Work out the finished part from the listing and answer in its coordinate system (mm). Face numbers are marked on the shaded views. A direction names the side the tool comes from. Round coordinates to 2 decimals unless told otherwise and drop trailing zeros. Loops run counter-clockwise (first coordinate to the right, second up) from the corner with the lowest first, then second, coordinate; pieces in that order, holes last. Notation, with made-up numbers: (13, 4.25) - (59, 4.25) arc R23 cw to (59, 31.25) - close; hole circle Ø11 at (-38.5, 6). An arc over 180 degrees is marked (long way). Answer as CSV lines item,"result". Start each with the question number.
Q1. Straight lines are drawn through the part: L1, parallel to Z at x = 0, y = 2.5; L2, parallel to Y at x = 5, z = -12.5; L3, parallel to Z at x = -20.5, y = 3. For each, find the intervals that lie inside material, in ascending order. Write a range as [from, to].
Q2. Section C-C on y = 12.75 is taken. Write down the section's boundary in (x, z).
Q3. For the marked faces 1 and 2, determine the directions among +Z, -Z, +X, -X, +Y, -Y from which every point of the face is accessible in a straight line to the end or side of a thin tool.
Q4. Section A-A on z = 0 is taken. Write down the section's boundary in (x, y), then the cut area to 3 significant figures.
Q5. The mould has two halves that part along Z. Classify the marked faces 3, 4 and 5: +Z half, -Z half, draft (parallel to the pull), parting line (faces both ways), or undercut.
Q6. Each of these flat-tipped pins is pushed along its axis until it touches: pin 1 Ø6 at (x, y) = (-10, 9) entering from -Z; pin 2 Ø5 at (x, y) = (-9.5, 3.5) entering from +Z; pin 3 Ø2.5 at (x, z) = (-16.5, 0) entering from -Y; pin 4 Ø3 at (x, y) = (-11, 6) entering from +Z. Where does it stop, or does it pass through?
Q7. Section B-B on x = 0 is taken. Write down the section's boundary in (y, z), then the cut area to 3 significant figures.
Q8. Section D-D on z = -16.5 is taken. Write down the section's boundary in (x, y).
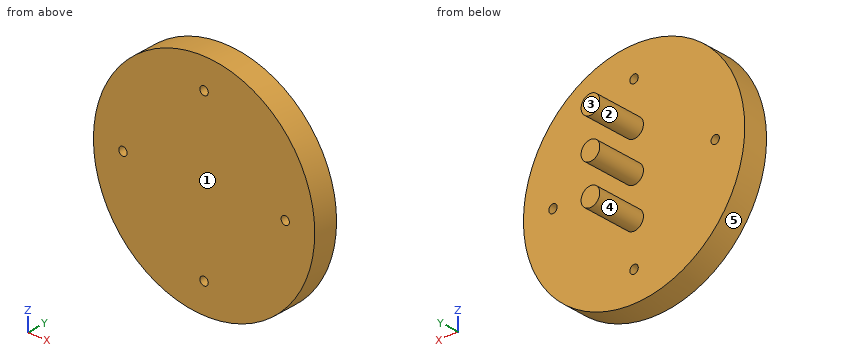
Autodesk Inventor part; units mm, degrees
ref_plane "YZ Plane" through (0, 0, 0) normal (1, 0, 0) x (0, 1, 0)
ref_plane "XZ Plane" through (0, 0, 0) normal (0, 1, 0) x (-1, 0, 0)
ref_plane "XY Plane" through (0, 0, 0) normal (0, 0, 1) x (1, 0, 0)
sketch "Sketch1" plane through (0, 0, 0) normal (0, 1, 0) x (-1, 0, 0)
  circle A0 centre (0, 0) radius 22.5
  dimension "d0" = 45
extrude "Extrusion1" add sketch "Sketch1" along normal blind 5
sketch "Sketch2" plane through (0, 5, 0) normal (0, 1, 0) x (1, 0, 0)
  line L0 (0, 0) -> (0, 8) construction
  line L1 (0, 0) -> (0, -8) construction
  circle A0 centre (0, 8) radius 1.9
  circle A1 centre (0, 0) radius 1.9
  circle A2 centre (0, -8) radius 1.9
  dimension "d3" = 8
  dimension "d4" = 8
  dimension "d5" = 3.8
  dimension "d6" = 3.8
  dimension "d7" = 3.8
extrude "Extrusion2" add sketch "Sketch2" along normal blind 10
sketch "Sketch7" plane through (0, 0, 0) normal (0, -1, 0) x (1, 0, 0)
  circle A0 centre (0, 0) radius 16.5 construction
  circle A1 centre (0, 16.5) radius 0.85
  circle A2 centre (16.5, 0) radius 0.85
  circle A3 centre (-16.5, 0) radius 0.85
  circle A4 centre (0, -16.5) radius 0.85
  dimension "d42" = 33
  dimension "d43" = 1.7
  dimension "d44" = 1.7
  dimension "d45" = 1.7
  dimension "d46" = 1.7
extrude "Extrusion6" cut sketch "Sketch7" against normal blind 5
properties part number "Motor Mount Barebones"
Findings:
1,L1,"z = [-22.5, -17.35], [-15.65, 15.65], [17.35, 22.5]"
1,L2,"y = [0, 5]"
1,L3,"z = [-9.27, 9.27]"
2,outline,"circle Ø3.8 at (0, -8); circle Ø3.8 at (0, 0); circle Ø3.8 at (0, 8)"
3,face 1,"+Z, -Z, +X, -X, -Y"
3,face 2,"+Y"
4,outline,"(-22.5, 0) - (-17.35, 0) - (-17.35, 5) - (-22.5, 5) - close; (-15.65, 0) - (15.65, 0) - (15.65, 5) - (1.9, 5) - (1.9, 15) - (-1.9, 15) - (-1.9, 5) - (-15.65, 5) - close; (17.35, 0) - (22.5, 0) - (22.5, 5) - (17.35, 5) - close"
4,area,"246 mm^2"
5,face 3,"draft"
5,face 4,"undercut"
5,face 5,"parting line"
6,pin 1,"passes through"
6,pin 2,"stops at z = 21.38"
6,pin 3,"stops at y = 0"
6,pin 4,"stops at z = 20.21"
7,outline,"(0, -22.5) - (5, -22.5) - (5, -17.35) - (0, -17.35) - close; (0, -15.65) - (5, -15.65) - (5, -9.9) - (15, -9.9) - (15, -6.1) - (5, -6.1) - (5, -1.9) - (15, -1.9) - (15, 1.9) - (5, 1.9) - (5, 6.1) - (15, 6.1) - (15, 9.9) - (5, 9.9) - (5, 15.65) - (0, 15.65) - close; (0, 17.35) - (5, 17.35) - (5, 22.5) - (0, 22.5) - close"
7,area,"322 mm^2"
8,outline,"(-15.3, 0) - (-0.85, 0) - (-0.85, 5) - (-15.3, 5) - close; (0.85, 0) - (15.3, 0) - (15.3, 5) - (0.85, 5) - close"
